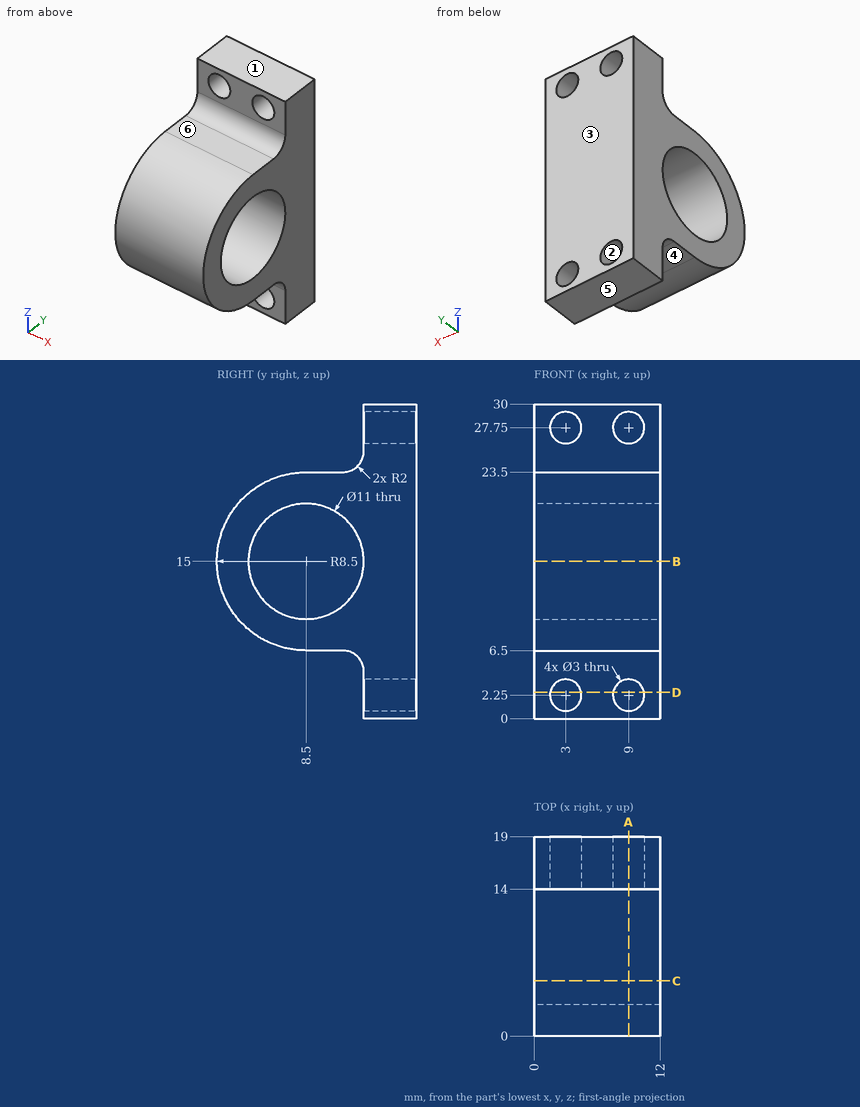
Could you check a few things on this drawing? It's one solid part, dimensions in mm from its lowest x, y, z. A direction names the side the tool comes from. Coordinates: 2 decimals unless noted, no trailing zeros. Order: outer loops, then holes, each group sorted by start corner. A loop starts at its lowest first (then second) coordinate and runs counter-clockwise, first axis right, second up. Notation, with made-up numbers: (-39.75, 44.25) - (-18.75, 44.25) arc R25 ccw to (-18.75, 61.25) - close; hole circle Ø8 at (72.5, 5). An arc over 180 degrees is marked (long way). Answer as a JSON object with one key per item and string values. Group by question number.
Q1. Imagine slicing it at A-A (x = 9). Please give me the cut outline in (y, z).
Q2. We'd pull the mould along Z, two halves only. Please class the marked faces 1, 2 and 3: +Z half, -Z half, draft (parallel to the pull), parting line (faces both ways), or undercut.
Q3. Imagine slicing it at B-B (z = 15). Please give me the cut outline in (x, y), and give its area (3 significant figures).
Q4. Imagine slicing it at D-D (z = 2.5). Please give me the cut outline in (x, y).
Q5. I need wall thicknesses on line 1 (X direction, y = 17.15, z = 2.25); line 2 (Y direction, x = 4.5, z = 15); line 3 (Z direction, x = 8.25, y = 8.25). Which ranges of each line are inside material? Lowest first, please. Write a range as from..to.
Q6. Imagine slicing it at C-C (y = 5.25). Please give me the cut outline in (x, z), and give its area (3 significant figures).
Q7. Will these pins go through, and if not, where does the flat tip stop? P1, Ø2, axis at x = 4.5, z = 25.5, coming from the -Y side; P2, Ø1.3, axis at x = 5.5, z = 27.5, coming from the -Y side; P3, Ø4, axis at x = 5, y = 10.5, coming from the +Z side.
Q8. On a 3-axis mill with a long thin cutter (end or side, diameter ignored), from which of +Z, -Z, +X, -X, +Y, -Y can I reach the whole of each face in a straight line? I mean the marked faces 4, 5 and 6. Say none if no direction works.
Determined:
{
 "1": {"outline": "(8.5, 6.5) - (12, 6.5) arc R2 cw to (14, 4.5) - (14, 3.75) - (19, 3.75) - (19, 26.25) - (14, 26.25) - (14, 25.5) arc R2 cw to (12, 23.5) - (8.5, 23.5) arc R8.5 ccw to start; (14, 0) - (19, 0) - (19, 0.75) - (14, 0.75) - close; (14, 29.25) - (19, 29.25) - (19, 30) - (14, 30) - close; hole circle Ø11 at (8.5, 15)"},
 "2": {"face 1": "+Z half", "face 2": "undercut", "face 3": "draft"},
 "3": {"outline": "(0, 0) - (12, 0) - (12, 3) - (0, 3) - close; (0, 14) - (12, 14) - (12, 19) - (0, 19) - close", "area": "96.0 mm2"},
 "4": {"outline": "(0, 14) - (1.52, 14) - (1.52, 19) - (0, 19) - close; (4.48, 14) - (7.52, 14) - (7.52, 19) - (4.48, 19) - close; (10.48, 14) - (12, 14) - (12, 19) - (10.48, 19) - close"},
 "5": {"line 1": "x = 0..1.5, 4.5..7.5, 10.5..12", "line 2": "y = 0..3, 14..19", "line 3": "z = 6.5..9.51, 20.49..23.5"},
 "6": {"outline": "(0, 7.15) - (12, 7.15) - (12, 10.56) - (0, 10.56) - close; (0, 19.44) - (12, 19.44) - (12, 22.85) - (0, 22.85) - close", "area": "82.0 mm2"},
 "7": {"P1": "stops at y = 13.73", "P2": "stops at y = 14", "P3": "stops at z = 23.56"},
 "8": {"face 4": "-Z, +X, -X, -Y", "face 5": "-Z, +X, -X, +Y, -Y", "face 6": "+Z, +X, -X, -Y"}
}
